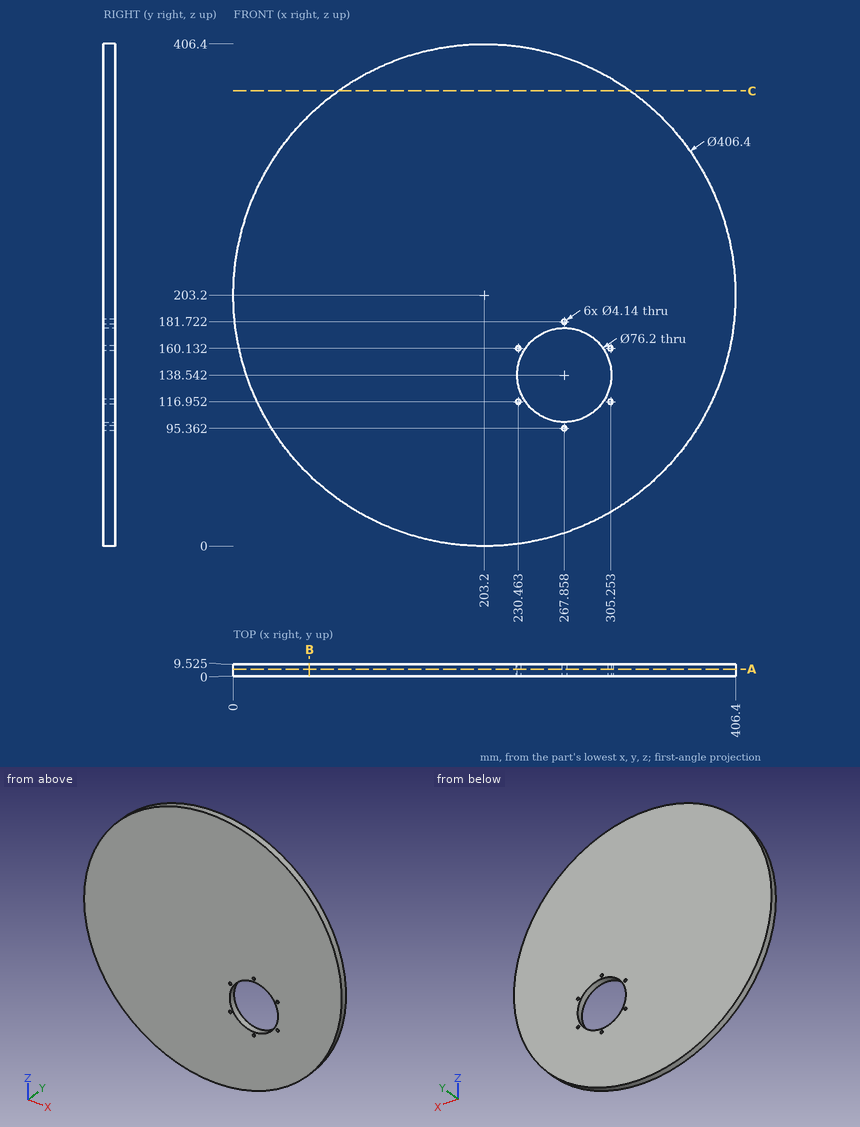
Check sheet for the drawn part. Datum: minimum x, y, z corner. Units: mm. Round coordinates to 2 decimals unless told otherwise and drop trailing zeros. Order: outer loops, then holes, each group sorted by start corner. A loop starts at its lowest first (then second) coordinate and runs counter-clockwise, first axis right, second up.
1) Scan lines: line 1 (Z direction, x = 205.5, y = 5.25); line 2 (X direction, y = 7.5, z = 103.5) (1 decimal); line 3 (Z direction, x = 254, y = 4.75). Record each from-to range of solid material in increasing order.
2) Section check C-C (z = 368.5). Record the boundary of the cut face in (x, y) (1 decimal), and give its area (3 significant figures).
3) Section check A-A (y = 5.5). Record the boundary of the cut face in (x, z).
4) Section check B-B (x = 61.5). Record the boundary of the cut face in (y, z) (1 decimal).
5) Go/stop test with flat-tipped pins: pin 1 Ø2 at (x, y) = (293, 2) entering from -Z; pin 2 Ø3 at (x, y) = (96.5, 5.5) entering from +Z. Record where each tip stops, or that it passes through.
Result:
1. line 1: z = 0.01 to 406.39
1. line 2: x = 26.1 to 252.9, 282.8 to 380.3
1. line 3: z = 6.45 to 103.05, 174.03 to 399.95
2. outline: (85, 0) - (321.4, 0) - (321.4, 9.5) - (85, 9.5) - close
2. area: 2,250 mm2
3. outline: circle Ø406.4 at (203.2, 203.2); hole circle Ø4.14 at (230.46, 116.95); hole circle Ø4.14 at (230.46, 160.13); hole circle Ø76.2 at (267.86, 138.54); hole circle Ø4.14 at (267.86, 95.36); hole circle Ø4.14 at (267.86, 181.72); hole circle Ø4.14 at (305.25, 116.95); hole circle Ø4.14 at (305.25, 160.13)
4. outline: (0, 57.6) - (9.5, 57.6) - (9.5, 348.8) - (0, 348.8) - close
5. pin 1: stops at z = 20.43
5. pin 2: stops at z = 377.05
